Part model, mm, in its own coordinate system. Face numbers are marked on the shaded views. A direction names the side the tool comes from. Round coordinates to 2 decimals unless told otherwise and drop trailing zeros. Write each loop counter-clockwise with the first axis right and the second up, starting at its lowest first coordinate (ties: lowest second). Pieces come first, ordered by that corner, then holes. Notation, with made-up numbers: (49.5, 13) -> (84.5, 13) arc R9 cw to (84.5, 24) -> close; hole circle Ø1 at (18, 9.25). An arc over 180 degrees is marked (long way). Return JSON: item names as keys, results as strings. Group by question number.
```python
from build123d import *

# Parameters (mm, degrees)
SKETCH4_W           = 62.83623107
SKETCH4_H           = 84.722256574
BOSS_EXTRUDE2_DEPTH = 50
CUT_EXTRUDE2_DEPTH  = 80
CUT_EXTRUDE3_DEPTH  = 80
CUT_EXTRUDE5_DEPTH  = 80
CUT_EXTRUDE6_DEPTH  = 3
CUT_EXTRUDE8_DEPTH  = 80


with BuildPart() as part:
    # Sketch4 → Boss-Extrude2 (new body)
    with BuildSketch(Plane.XY):
        Rectangle(SKETCH4_W, SKETCH4_H)
    extrude(amount=BOSS_EXTRUDE2_DEPTH)

    # Sketch5 → Cut-Extrude2 (cut)
    with BuildSketch(Plane(origin=(31.418115535, 0, 0), x_dir=(0, 0, -1), z_dir=(1, 0, 0))):
        Polygon((-31.846034257, 38.728174008), (-31.846034257, 42.361128287), (-50, 42.361128287), (-50, -42.361128287), (-30.898434646, -42.361128287), (-30.898434646, -37.982426726), (-46.322270236, 2.38891709), align=None)
    extrude(amount=-CUT_EXTRUDE2_DEPTH, mode=Mode.SUBTRACT)

    # Sketch6 → Cut-Extrude3 (cut)
    with BuildSketch(Plane(origin=(31.418115535, 0, 0), x_dir=(0, 0, -1), z_dir=(1, 0, 0))):
        Polygon((-29.655383969, 42.361128287), (-29.655383969, 38.722554473), (-8.776416022, 3.750158878), (-28.328453067, -38.117745), (-28.328453067, -42.361128287), (-27.677514405, -46.625913761), (16.839811583, -52.045359618), (10.267667228, 27.190343951), (3.73953172, 54.484047391), align=None)
    extrude(amount=-CUT_EXTRUDE3_DEPTH, mode=Mode.SUBTRACT)

    # Sketch7 → Cut-Extrude5 (cut)
    with BuildSketch(Plane.ZY.offset(31.418115535)):
        with BuildLine():
            ThreePointArc((13.228873585, 11.208051798), (10.417703783, 4.563945687), (11.71087014, -2.533556863))
            ThreePointArc((11.71087014, -2.533556863), (0.747619784, 5.632177302), (13.228873585, 11.208051798))
        make_face()
    extrude(amount=-CUT_EXTRUDE5_DEPTH, mode=Mode.SUBTRACT)

    # Sketch8 → Cut-Extrude6 (cut)
    with BuildSketch(Plane(origin=(31.418115535, 0, 0), x_dir=(0, 0, -1), z_dir=(1, 0, 0))):
        Polygon((-30.111598921, 36.817435747), (-42.735074125, 2.19595341), (-30.111598921, -36.694083179), (-29.289064541, -37.07820135), (-12.845557678, 2.19595341), align=None)
    extrude(amount=-CUT_EXTRUDE6_DEPTH, mode=Mode.SUBTRACT)

    # Sketch9 → Cut-Extrude8 (cut)
    with BuildSketch(Plane(origin=(0, 0, 29.655383969), x_dir=(-1, 0, 0), z_dir=(0, 0, -1))):
        Polygon((19.869908303, 42.361128287), (19.869908303, 38.722554473), (19.869908303, 5.586987563), (19.869908303, -4.186945454), (19.869908303, -38.208459621), (19.869908303, -42.059759196), (19.869908303, -47.026854784), (41.256673117, -49.585938288), (42.081255469, -21.197702537), (42.081255469, 12.428184914), (37.482224788, 37.513066745), (31.418115535, 49.4837873), align=None)
    extrude(amount=-CUT_EXTRUDE8_DEPTH, mode=Mode.SUBTRACT)


solid = part.part
```
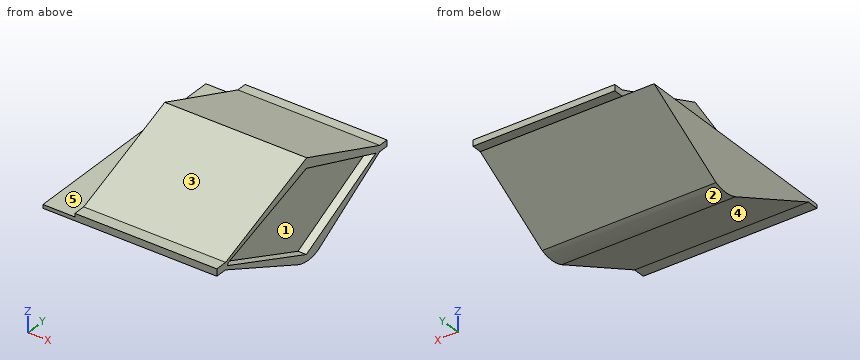
Item 1: Wall check: L1, parallel to X at y = 23, z = 35.5; L2, parallel to X at y = 0.5, z = 15; L3, parallel to Z at x = 0, y = 14. Give the ranges that are in metal, low to high.
Item 2: Which spindle directions (+Z, -Z, +X, -X, +Y, -Y) get a long thin tool onto all of the face, cutting with end or side? Do the marked faces 4 and 5. Say none if no direction does.
Item 3: Cut at C-C (y = 21). Write the cut outline in (x, z).
Item 4: Flat gauge pins, fed straight in: P1, Ø8, axis at y = 6, z = 20, coming from the +X side; P2, Ø1, axis at y = -12, z = 40, coming from the -X side; P3, Ø2, axis at x = -0.5, y = -41, coming from the +Z side; P4, Ø2, axis at y = 20.5, z = 17.5, coming from the -X side. Where does each tip first touch, or does it go through?
Item 5: Cut at B-B (z = 41). Write the cut outline in (x, y), then the cut area to 3 significant figures.
Item 6: Cut at D-D (x = -25). Write the cut outline in (y, z), then the cut area to 3 significant figures.
Item 7: Two-plate mould, pull along Y, no slides. Class the marked faces 1, 2 and 3: released by +Y, released by -Y, zero draft, split by the parting line, or undercut.
Item 8: Cut at A-A (x = 27). Write the cut outline in (y, z), then the cut area to 3 significant figures.
Checks:
{
 "1": {"L1": "x = -19.87 to 31.42", "L2": "x = -31.42 to 28.42", "L3": "z = 14.9 to 41.7"},
 "2": {"face 4": "-Z, +X, -X, -Y", "face 5": "+Z, -X, +Y, -Y"},
 "3": {"outline": "(-31.42, 19.07) -> (31.42, 19.07) -> (31.42, 22.22) -> (28.42, 22.22) -> (28.42, 35.88) -> (31.42, 35.88) -> (31.42, 38.91) -> (-19.87, 38.91) -> (-19.87, 29.66) -> (-31.42, 29.66) -> close"},
 "4": {"P1": "stops at x = 28.42", "P2": "stops at x = -19.87", "P3": "stops at z = 30.9", "P4": "passes through"},
 "5": {"outline": "(-19.87, -11.54) -> (31.42, -11.54) -> (31.42, -3.15) -> (28.42, -3.15) -> (28.42, 6.95) -> (31.42, 6.95) -> (31.42, 15.75) -> (-19.87, 15.75) -> close", "area": "1,370 mm2"},
 "6": {"outline": "(-42.36, 28.33) -> (-38.12, 28.33) -> (-1.77, 11.35) arc R12.6 ccw to (7.92, 11.27) -> (38.72, 29.66) -> (-42.36, 29.66) -> close", "area": "830 mm2"},
 "7": {"face 1": "undercut", "face 2": "split by the parting line", "face 3": "released by -Y"},
 "8": {"outline": "(-42.36, 28.33) -> (-38.12, 28.33) -> (-1.77, 11.35) arc R12.6 ccw to (7.92, 11.27) -> (38.72, 29.66) -> (42.36, 29.66) -> (42.36, 31.85) -> (38.73, 31.85) -> (2.39, 46.32) -> (-37.98, 30.9) -> (-42.36, 30.9) -> close", "area": "1,550 mm2"}
}
